```python
from build123d import *

# Parameters (mm, degrees)
F1_DEPTH = 65.532
F2_R     = 1.905
F3_DEPTH = 52.671675


with BuildPart() as f1:
    # F0 (on Front) → F1 (new body)
    with BuildSketch(Plane.XZ):
        Polygon((34.087103, 10.257693), (34.087103, 0), (41.662011, 0), (41.662011, 10.257693), (62.177397, 10.257693), (62.177397, 0), (76.695979, 0), (76.695979, 7.417101), (88.058345, 7.417101), (88.058345, 18.463846), (69.752306, 32.351185), (50.183784, 32.351185), (46.080712, 24.460651), (36.29645, 18.463846), (25.249707, 18.463846), (28.090296, 10.257693), align=None)
    extrude(amount=F1_DEPTH)

    # F2 (on face) → F3 (cut, through all)
    with BuildSketch(Plane(origin=(41.056729, 0, 54.12024), x_dir=(0.796691, 0, -0.604386), z_dir=(0.604386, 0, 0.796691))):
        with Locations((47.507229, -32.766)):
            Circle(F2_R)
    extrude(amount=-F3_DEPTH, mode=Mode.SUBTRACT)


solid = f1.part
```
The model under review builds one solid part; all positions refer to its coordinate system, in mm. A direction names the side the tool comes from. Give positions to 0.01 mm unless a question says otherwise; leave off trailing zeros. Write each loop counter-clockwise with the first axis right and the second up, starting at its lowest first coordinate (ties: lowest second). Pieces come first, ordered by that corner, then holes. Notation, with made-up numbers: M 32,49.25 L 56,49.25 A11 ccw 56,64.25 Z; hole C 61,62.25 d10. An arc over 180 degrees is marked long. Write item = value, one per line. Start each with the question number.
Q1. Machinability: for faces 1 (the face through (31, -32, 10.258)), 2 (the face through (31, -32, 18.464)), 3 (the face through (41.662, -32, 5)), 4 (the face through (88.058, -32, 13)), 5 (the face through (76.696, -32, 4)), which of the approach directions +Z, -Z, +X, -X, +Y, -Y give a long, thin tool a straight path to every point of the face, cutting with its end or side? Answer none if there is none.
Q2. Clearance check with flat-ended pins moving along their axes: pin 1 (2 mm diameter, centred on y = -33.5, z = 5.5, fed in from +X); pin 2 (12 mm diameter, centred on x = 80, z = 21.5, fed in from +Y); pin 3 (8 mm diameter, centred on y = -41.5, z = 7, fed in from -X); pin 4 (5 mm diameter, centred on x = 31, y = -39, fed in from -Z). State where each tip first meets the part, or that it passes through.
Q3. Mouldability with a two-part tool opening along Y and no side actions: class faces 6 (the face through (56, -65.532, 16)), 7 (the face through (71.31, -33.5, 12.49)), 8 (the face through (69, -32, 0)), 9 (the face through (56, 0, 16)) as released by +Y, released by -Y, zero draft, split by the parting line, or undercut.
Q4. We need section B-B (x = 83). State the section outline as (y, z) points, plus the area to 3 significant figures.
Q5. For line 1 (X direction, y = -24, z = 10); line 2 (X direction, y = -44, z = 6.5); line 3 (Z direction, x = 54, y = -18), list the stretches that pass through material, from the lowest coordinate up.
Q6. We need section C-C (z = 29). State the section outline as (x, y) points.
Q7. We need section A-A (y = -37). State the section outline as (x, z) points.
Result set:
q1.face_1 = -Z, -X, +Y, -Y
q1.face_2 = +Z, -X, +Y, -Y
q1.face_3 = -Z, +Y, -Y
q1.face_4 = +Z, -Z, +X, +Y, -Y
q1.face_5 = -Z, +X, +Y, -Y
q2.pin_1 = 76.7
q2.pin_2 = 0
q2.pin_3 = 27.83
q2.pin_4 = 10.26
q3.face_6 = released by -Y
q3.face_7 = undercut
q3.face_8 = zero draft
q3.face_9 = released by +Y
q4.outline = M -65.53,7.42 L 0,7.42 L 0,22.3 L -65.53,22.3 Z
q4.area = 975 mm2
q5.line_1 = 34.09 to 41.66, 62.18 to 88.06
q5.line_2 = 34.09 to 41.66, 62.18 to 76.7
q5.line_3 = 10.26 to 32.35
q6.outline = M 48.44,-65.53 L 74.17,-65.53 L 74.17,0 L 48.44,0 Z
q7.outline = M 25.25,18.46 L 28.09,10.26 L 34.09,10.26 L 34.09,0 L 41.66,0 L 41.66,10.26 L 62.18,10.26 L 62.18,0 L 76.7,0 L 76.7,7.42 L 88.06,7.42 L 88.06,18.46 L 69.75,32.35 L 50.18,32.35 L 46.08,24.46 L 36.3,18.46 Z
